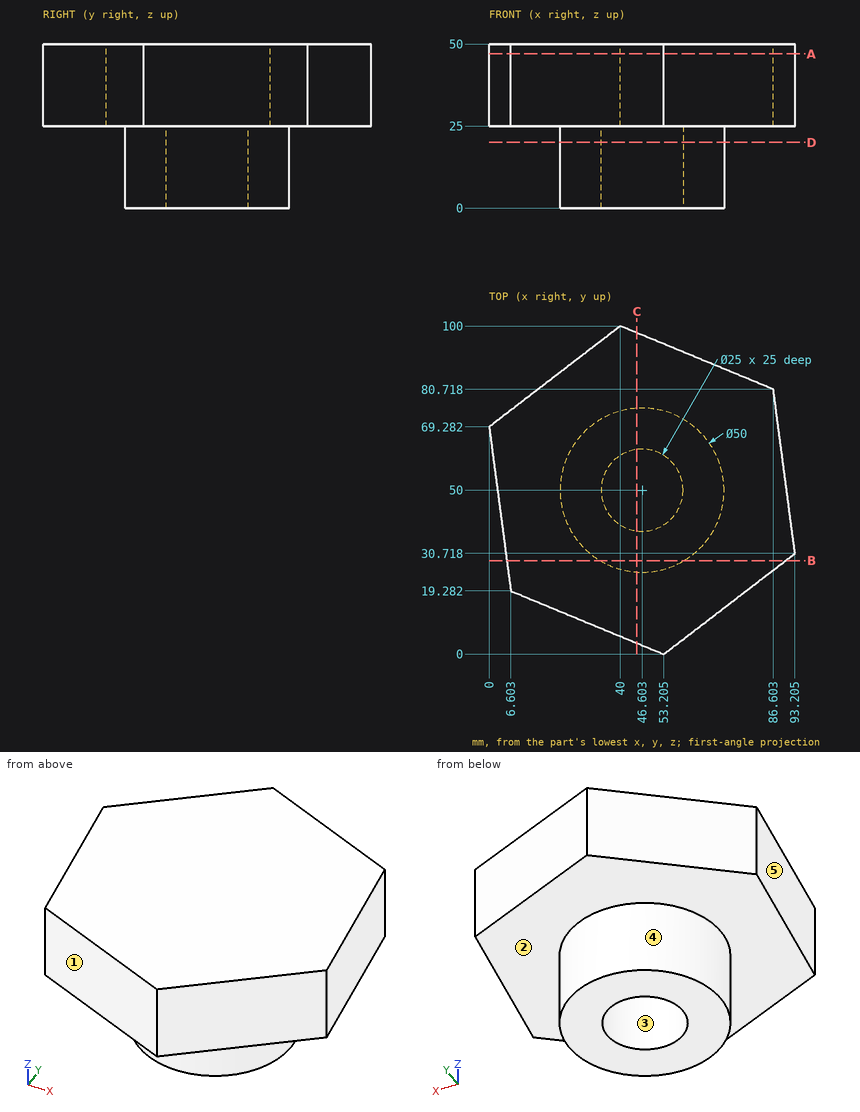
The figure shows three views and two pictorial views of one solid part (mm, origin at its lowest corner). Answer the questions. A direction names the side the tool comes from. Round coordinates to 2 decimals unless told otherwise and drop trailing zeros. Loops run counter-clockwise (first coordinate to the right, second up) from the corner with the lowest first, then second, coordinate; pieces in that order, holes last. Notation, with made-up numbers: (-19.75, -38.75) - (28.25, -38.75) arc R10 cw to (28.25, -32.75) - close; hole circle Ø5 at (31, 34.5). An arc over 180 degrees is marked (long way). One line per question, with ' | ' between items. Start each with the question number.
Q1. Section D-D on z = 20 is taken. Give the vertices of the cut face in (x, y), plus the area to 3 significant figures.
Q2. For the marked faces 1 and 2, determine the directions among +Z, -Z, +X, -X, +Y, -Y from which every point of the face is accessible in a straight line to the end or side of a thin tool.
Q3. Section B-B on y = 28.5 is taken. Give the vertices of the cut face in (x, z) (1 decimal).
Q4. Section C-C on x = 45 is taken. Give the vertices of the cut face in (y, z) (1 decimal), plus the area to 3 significant figures.
Q5. Flat-ended cylindrical pins translate along their axes: pin 1 (3 mm diameter, centred on y = 35.5, z = 32.5, fed in from +X); pin 2 (4 mm diameter, centred on y = 79, z = 22.5, fed in from -X); pin 3 (1 mm diameter, centred on x = 16, z = 40.5, fed in from -Y); pin 4 (2 mm diameter, centred on x = 70, y = 37, fed in from -Z). Find the tip coordinate at first contact, or state that the pin passes through.
Q6. Find the intervals of material crossed by L1, parallel to Z at x = 64, y = 77; L2, parallel to X at y = 48, z = 3; L3, parallel to X at y = 31.5, z = 10 (1 decimal), in increasing order.
Q7. For a pull along X with two mould halves and no side action, classify the marked faces 3, 4 and 5 as +X half, -X half, draft (parallel to the pull), parting line (faces both ways), or undercut.
Q8. Section A-A on z = 47 is taken. Give the vertices of the cut face in (x, y) (1 decimal).
Established:
1) outline: circle Ø50 at (46.6, 50); hole circle Ø25 at (46.6, 50) | area: 1,470 mm²
2) face 1: +Z, -Z, -X, -Y | face 2: -Z
3) outline: (5.4, 25) - (33.8, 25) - (33.8, 0) - (59.4, 0) - (59.4, 25) - (90.3, 25) - (90.3, 50) - (5.4, 50) - close
4) outline: (3.4, 25) - (25.1, 25) - (25.1, 0) - (37.6, 0) - (37.6, 25) - (62.4, 25) - (62.4, 0) - (74.9, 0) - (74.9, 25) - (97.9, 25) - (97.9, 50) - (3.4, 50) - close | area: 2,990 mm²
5) pin 1: x = 92.77 | pin 2: through | pin 3: y = 15.19 | pin 4: z = 25
6) L1: 25 to 50 | L2: 21.68 to 34.26, 58.94 to 71.52 | L3: 29.8 to 63.4
7) face 3: undercut | face 4: parting line | face 5: -X half
8) outline: (0, 69.3) - (6.6, 19.3) - (53.2, 0) - (93.2, 30.7) - (86.6, 80.7) - (40, 100) - close
